Design review of the part built by this model. Coordinates are the model's own, in mm. A direction names the side the tool comes from. Coordinates: 2 decimals unless noted, no trailing zeros. Loops run counter-clockwise (first coordinate to the right, second up) from the corner with the lowest first, then second, coordinate; pieces in that order, holes last. Notation, with made-up numbers: M 1,44.5 L 57,44.5 A22 cw 57,65.5 Z; hole C 44.5,-14 d8. An arc over 180 degrees is marked long. Answer as CSV lines item,"result". Start each with the question number.
from build123d import *

# Parameters (mm, degrees)
SKETCH1_W                  = 30
SKETCH1_H                  = 25
BOSS_EXTRUDE1_DEPTH        = 14
F_3_2_3_2_DIAMETER_HOLE1_D = 3.2
SKETCH5_W                  = 7
SKETCH5_H                  = 20
CUT_EXTRUDE1_DEPTH         = 10
SKETCH6_W                  = 10
SKETCH6_H                  = 25
CUT_EXTRUDE2_DEPTH         = 5
CHAMFER1_SIZE              = 1
SKETCH7_W                  = 14
SKETCH7_H                  = 25
BOSS_EXTRUDE2_DEPTH        = 23


with BuildPart() as part:
    # Sketch1 → Boss-Extrude1 (new body)
    with BuildSketch(Plane(origin=(0, 0, 0), x_dir=(1, 0, 0), z_dir=(0, 1, 0))):
        with Locations((15, 0)):
            Rectangle(SKETCH1_W, SKETCH1_H)
    extrude(amount=BOSS_EXTRUDE1_DEPTH)

    # Ø3.2 (3.2) Diameter Hole1 (through all)
    with Locations(Plane(origin=(0, 14, 0), x_dir=(1, 0, 0), z_dir=(0, 1, 0))):
        with Locations((5, 7.5), (5, -7.5)):
            Hole(F_3_2_3_2_DIAMETER_HOLE1_D / 2)

    # Sketch5 → Cut-Extrude1 (cut)
    with BuildSketch(Plane(origin=(0, 14, 0), x_dir=(1, 0, 0), z_dir=(0, 1, 0))):
        with Locations((20, 0)):
            Rectangle(SKETCH5_W, SKETCH5_H)
    extrude(amount=-CUT_EXTRUDE1_DEPTH, mode=Mode.SUBTRACT)

    # Sketch6 → Cut-Extrude2 (cut)
    with BuildSketch(Plane(origin=(0, 14, 0), x_dir=(1, 0, 0), z_dir=(0, 1, 0))):
        with Locations((5, 0)):
            Rectangle(SKETCH6_W, SKETCH6_H)
    extrude(amount=-CUT_EXTRUDE2_DEPTH, mode=Mode.SUBTRACT)

    # Chamfer1
    chamfer1_edges = [part.edges().sort_by_distance(p)[0] for p in [
        (0, 9, 0),
    ]]
    chamfer(chamfer1_edges, length=CHAMFER1_SIZE)

    # Sketch7 → Boss-Extrude2 (add)
    with BuildSketch(Plane.XZ):
        with Locations((23, 0)):
            Rectangle(SKETCH7_W, SKETCH7_H)
    extrude(amount=BOSS_EXTRUDE2_DEPTH)


solid = part.part
Item 1: Add section A-A (x = 5). Give the boundary of the cut face in (y, z), plus the area to 3 significant figures.
Item 2: Add section D-D (z = 5). Give the boundary of the cut face in (x, y), plus the area to 4 significant figures.
Item 3: For faces 4 (the face through (16, -11, 0)), 5 (the face through (5, 9, 0)), 6 (the face through (20, 9, -10)), list the 3-axis set-ups (+Z, -Z, +X, -X, +Y, -Y) from which the entire face can be reached by the end or side of a thin tool; tool diameter is ignored.
Item 4: For pin 1 (1.5 mm diameter, centred on y = 12.5, z = 3.5, fed in from -X); pin 2 (2 mm diameter, centred on x = 3.5, z = -0.5, fed in from -Y); pin 3 (5 mm diameter, centred on x = 4, z = 4, fed in from +Y); pin 4 (3 mm diameter, centred on x = 5, z = 7.5, fed in from -Y), all flat-tipped, find the tip position at first contact; note any pin that passes through.
Item 5: Mouldability with a two-part tool opening along X and no side actions: class faces 1 (the face through (15, 14, 0)), 2 (the face through (10, 12, 0)), 3 (the face through (20, 4, 0)) as released by +X, released by -X, zero draft, split by the parting line, or undercut.
Item 6: Add section B-B (z = 7.5). Give the boundary of the cut face in (x, y).
Item 7: Add section C-C (y = 7). Give the boundary of the cut face in (x, z).
Item 8: For line 1 along Z through (x, y) = (5, 5); line 2 along X through (y, z) = (5.5, 7.5); line 3 along X through (y, z) = (10, 4.75), list the stretches that pass through material, from the lowest coordinate up. Write a range as from..to.
Response:
1,outline,"M 0,-12.5 L 9,-12.5 L 9,-9.1 L 0,-9.1 Z; M 0,-5.9 L 9,-5.9 L 9,5.9 L 0,5.9 Z; M 0,9.1 L 9,9.1 L 9,12.5 L 0,12.5 Z"
1,area,"167 mm²"
2,outline,"M 0,0 L 16,0 L 16,-23 L 30,-23 L 30,14 L 23.5,14 L 23.5,4 L 16.5,4 L 16.5,14 L 10,14 L 10,9 L 1,9 L 0,8 Z"
2,area,"621.5 mm²"
3,face 4,"+Z, -Z, -X, -Y"
3,face 5,"+Z, -Z, -X, +Y"
3,face 6,"+Y"
4,pin 1,"x = 10"
4,pin 2,"y = 0"
4,pin 3,"y = 9"
4,pin 4,"through"
5,face 1,"zero draft"
5,face 2,"released by -X"
5,face 3,"undercut"
6,outline,"M 0,0 L 3.4,0 L 3.4,9 L 1,9 L 0,8 Z; M 6.6,0 L 16,0 L 16,-23 L 30,-23 L 30,14 L 23.5,14 L 23.5,4 L 16.5,4 L 16.5,14 L 10,14 L 10,9 L 6.6,9 Z"
7,outline,"M 0,-12.5 L 30,-12.5 L 30,12.5 L 0,12.5 Z; hole C 5,-7.5 d3.2; hole C 5,7.5 d3.2; hole M 16.5,-10 L 23.5,-10 L 23.5,10 L 16.5,10 Z"
8,line 1,"-12.5..-9.1, -5.9..5.9, 9.1..12.5"
8,line 2,"0..3.4, 6.6..16.5, 23.5..30"
8,line 3,"10..16.5, 23.5..30"
